The listing builds one solid part. Answer for the finished solid, in the listing's coordinates (mm). Coordinates: 2 decimals unless noted, no trailing zeros. Loops run counter-clockwise (first coordinate to the right, second up) from the corner with the lowest first, then second, coordinate; pieces in that order, holes last. Notation, with made-up numbers: (0, 80) - (39, 80) arc R13 cw to (39, 87) - close; hole circle Ø10 at (47.25, 64). An arc over 180 degrees is marked (long way). Return JSON: item names as keys, results as strings. Group by question number.
1. Find the intervals of material crossed by line 1 along Y through (x, z) = (1.35, 16); line 2 along Z through (x, y) = (-0.05, -25.65); line 3 along Z through (x, y) = (0, 27), in increasing order.
2. Section A-A (y = 10.5) is taken. Write down the section's boundary in (x, z), and give its area (3 significant figures).
3. Section B-B (z = 47.5) is taken. Write down the section's boundary in (x, y), and give its area (3 significant figures).
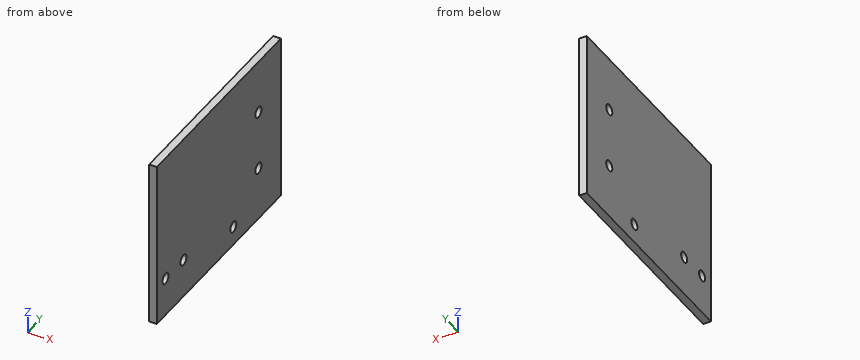
```python
from build123d import *

# Parameters (mm, degrees)
F0_W     = 3.175
F0_H     = 90
F1_DEPTH = 70
F3_D     = 4.4
F5_D     = 4.4
F5_DEPTH = 25
F5_TIP   = 1.3218933619


with BuildPart() as f1:
    # F0 (on Top) → F1 (new body)
    with BuildSketch(Plane.XY):
        Rectangle(F0_W, F0_H)
    extrude(amount=F1_DEPTH)

    # F3 (through all)
    with Locations(Plane(origin=(-1.5875, 0, 0), x_dir=(0, -1, 0), z_dir=(-1, 0, 0))):
        with Locations((-28.728, 47.5), (-28.728, 22.5)):
            Hole(F3_D / 2)

    # F5
    with Locations(Plane(origin=(-1.5875, 0, 0), x_dir=(0, -1, 0), z_dir=(-1, 0, 0))):
        with Locations((38.65, 16.272), (25.65, 16.272), (-10.5, 7.9375)):
            Hole(F5_D / 2, depth=F5_DEPTH)
            with Locations((0, 0, -(F5_DEPTH + F5_TIP / 2))):  # 118° drill point
                Cone(0, F5_D / 2, F5_TIP, mode=Mode.SUBTRACT)


solid = f1.part
```
The answers:
{
 "1": {"line 1": "y = -45 to -40.83, -36.47 to -27.83, -23.47 to 45", "line 2": "z = 0 to 14.07, 18.47 to 70", "line 3": "z = 0 to 21.14, 23.86 to 46.14, 48.86 to 70"},
 "2": {"outline": "(-1.59, 0) - (1.59, 0) - (1.59, 5.74) - (-1.59, 5.74) - close; (-1.59, 10.14) - (1.59, 10.14) - (1.59, 70) - (-1.59, 70) - close", "area": "208 mm2"},
 "3": {"outline": "(-1.59, -45) - (1.59, -45) - (1.59, 26.53) - (-1.59, 26.53) - close; (-1.59, 30.93) - (1.59, 30.93) - (1.59, 45) - (-1.59, 45) - close", "area": "272 mm2"}
}
